Check sheet for the modelled part. Datum: model origin and axes. Units: mm. Face numbers are marked on the shaded views. A direction names the side the tool comes from. Give positions to 0.01 mm unless a question says otherwise; leave off trailing zeros. Order: outer loops, then holes, each group sorted by start corner. A loop starts at its lowest first (then second) coordinate and runs counter-clockwise, first axis right, second up.
Item 1: Sectioned sample at D-D on x = 708. Record the boundary of the cut face in (y, z), and give its area (3 significant figures).
Item 2: Access from +Z, -Z, +X, -X, +Y, -Y to the whole of each face (thin tool, end or side, straight path). Record for the marked faces 1, 2 and 3.
Item 3: Sectioned sample at A-A on x = 144. Record the boundary of the cut face in (y, z), and give its area (3 significant figures).
Item 4: Release check for a two-part mould opening along Y. For the marked faces 4, 5, 6 and 7 record: released by +Y, released by -Y, zero draft, split by the parting line, or undercut.
Item 5: Material ranges on line 1 along Z through (x, y) = (1072, 76) (3 decimals); line 2 along Y through (x, z) = (584.5, 293.5); line 3 along Y through (x, z) = (560, -245.5), recorded low to high.
Item 6: Gauge pin test, flat ends, axial feed: P1, Ø6, axis at x = 123.5, z = 272.5, coming from the +Y side; P2, Ø20.5, axis at x = -667, z = 305.5, coming from the +Y side; P3, Ø6.5, axis at x = 1057.5, z = -48, coming from the +Y side. Record the tip position at first contact, or that the pin passes through.
Item 7: Sectioned sample at B-B on y = 381. Record the boundary of the cut face in (x, z), and give its area (3 significant figures).
Item 8: Sectioned sample at C-C on z = -208. Record the boundary of the cut face in (x, y).
from build123d import *

# Parameters (mm, degrees)
F1_DEPTH  = 1066.8
F2_W      = 101.6
F2_H      = 793.75
F2_R      = 14.2875
F3_DEPTH  = 139.7
F4_W      = 304.8
F4_H      = 222.25
F4_R      = 23.8125
F4_W_2    = 476.25
F5_DEPTH  = 25.4
F8_DEPTH  = 12.7
F9_W      = 101.6
F9_H      = 228.6
F9_R      = 7.14375
F10_DEPTH = 25.4


with BuildPart() as f1:
    # F0 (on Right) → F1 (new body, symmetric)
    with BuildSketch(Plane.YZ):
        with BuildLine():
            Line((476.25, 292.1), (-476.25, 292.1))
            ThreePointArc((-476.25, 292.1), (-498.7006403027, 282.8006403027), (-508, 260.35))
            Line((-508, 260.35), (-508, -260.35))
            ThreePointArc((-508, -260.35), (-513.5796158184, -273.8203841816), (-527.05, -279.4))
            Line((-527.05, -279.4), (-647.7, -279.4))
            Line((-647.7, -279.4), (-647.7, -292.1))
            Line((-647.7, -292.1), (-527.05, -292.1))
            ThreePointArc((-527.05, -292.1), (-504.5993596973, -282.8006403027), (-495.3, -260.35))
            Line((-495.3, -260.35), (-495.3, 260.35))
            ThreePointArc((-495.3, 260.35), (-489.7203841816, 273.8203841816), (-476.25, 279.4))
            Line((-476.25, 279.4), (476.25, 279.4))
            ThreePointArc((476.25, 279.4), (489.7203841816, 273.8203841816), (495.3, 260.35))
            Line((495.3, 260.35), (495.3, -260.35))
            ThreePointArc((495.3, -260.35), (504.5993596973, -282.8006403027), (527.05, -292.1))
            Line((527.05, -292.1), (647.7, -292.1))
            Line((647.7, -292.1), (647.7, -279.4))
            Line((647.7, -279.4), (527.05, -279.4))
            ThreePointArc((527.05, -279.4), (513.5796158184, -273.8203841816), (508, -260.35))
            Line((508, -260.35), (508, 260.35))
            ThreePointArc((508, 260.35), (498.7006403027, 282.8006403027), (476.25, 292.1))
        make_face()
    extrude(amount=F1_DEPTH, both=True)

    # F2 (on face) → F3 (join)
    with BuildSketch(Plane.XY.offset(292.1)):
        with Locations((901.7, -79.375)):
            Rectangle(F2_W, F2_H)
        with Locations((885.952, -234.95)):
            Circle(F2_R, mode=Mode.SUBTRACT)
        with Locations((885.952, 234.95)):
            Circle(F2_R, mode=Mode.SUBTRACT)
        with Locations((565.404, -79.375)):
            Rectangle(F2_W, F2_H)
        with Locations((581.152, -234.95)):
            Circle(F2_R, mode=Mode.SUBTRACT)
        with Locations((581.152, 234.95)):
            Circle(F2_R, mode=Mode.SUBTRACT)
    extrude(amount=F3_DEPTH)

    # F4 (on face) → F5 (join)
    with BuildSketch(Plane.XY.offset(292.1)):
        with Locations((-660.4, -358.775)):
            Rectangle(F4_W, F4_H)
        with Locations((-663.448, -381)):
            Circle(F4_R, mode=Mode.SUBTRACT)
        with Locations((238.125, -358.775)):
            Rectangle(F4_W_2, F4_H)
        with Locations((327.152, -381)):
            Circle(F4_R, mode=Mode.SUBTRACT)
        with Locations((238.125, 358.775)):
            Rectangle(F4_W_2, F4_H)
        with Locations((327.152, 381)):
            Circle(F4_R, mode=Mode.SUBTRACT)
        with Locations((-660.4, 358.775)):
            Rectangle(F4_W, F4_H)
        with Locations((-663.448, 381)):
            Circle(F4_R, mode=Mode.SUBTRACT)
    extrude(amount=F5_DEPTH)

    # F7 (on offset) → F8 (join)
    with BuildSketch(Plane.YZ.offset(1041.4)):
        Polygon((495.3, -260.35), (495.3, 260.35), (476.25, 279.4), (-476.25, 279.4), (-495.3, 260.35), (-495.3, -260.35), align=None)
    extrude(amount=F8_DEPTH)

    # F9 (on face) → F10 (join)
    with BuildSketch(Plane.YZ.offset(1054.1)):
        with Locations((50.8, 136.525)):
            Rectangle(F9_W, F9_H)
        with Locations((76.2, 85.852)):
            Circle(F9_R, mode=Mode.SUBTRACT)
        with Locations((76.2, 212.852)):
            Circle(F9_R, mode=Mode.SUBTRACT)
        with Locations((-50.8, 136.525)):
            Rectangle(F9_W, F9_H)
        with Locations((-76.2, 85.852)):
            Circle(F9_R, mode=Mode.SUBTRACT)
        with Locations((-76.2, 212.852)):
            Circle(F9_R, mode=Mode.SUBTRACT)
    extrude(amount=F10_DEPTH)


solid = f1.part
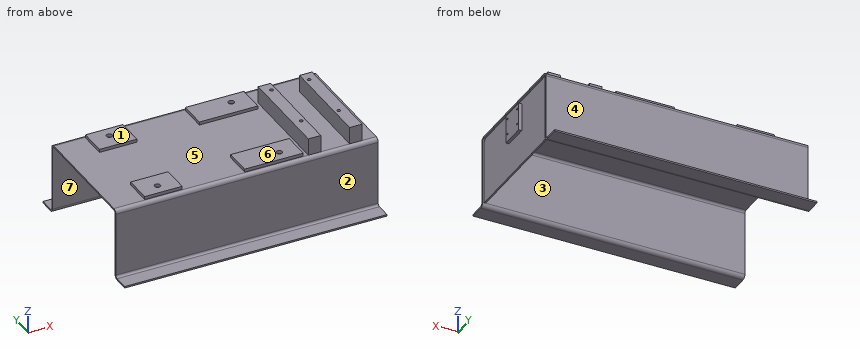
Report:
1. outline: (-647.7, -292.1) - (-527.05, -292.1) arc R31.75 ccw to (-495.3, -260.35) - (-495.3, 260.35) arc R19.05 cw to (-476.25, 279.4) - (476.25, 279.4) arc R19.05 cw to (495.3, 260.35) - (495.3, -260.35) arc R31.75 ccw to (527.05, -292.1) - (647.7, -292.1) - (647.7, -279.4) - (527.05, -279.4) arc R19.05 cw to (508, -260.35) - (508, 260.35) arc R31.75 ccw to (476.25, 292.1) - (-476.25, 292.1) arc R31.75 ccw to (-508, 260.35) - (-508, -260.35) arc R19.05 cw to (-527.05, -279.4) - (-647.7, -279.4) - close
1. area: 30,400 mm2
2. face 1: +Z, -X, +Y, -Y
2. face 2: +Z, +X, -X, -Y
2. face 3: -Z, -X
3. outline: (-647.7, -292.1) - (-527.05, -292.1) arc R31.75 ccw to (-495.3, -260.35) - (-495.3, 260.35) arc R19.05 cw to (-476.25, 279.4) - (476.25, 279.4) arc R19.05 cw to (495.3, 260.35) - (495.3, -260.35) arc R31.75 ccw to (527.05, -292.1) - (647.7, -292.1) - (647.7, -279.4) - (527.05, -279.4) arc R19.05 cw to (508, -260.35) - (508, 260.35) arc R31.75 ccw to (476.25, 292.1) - (469.9, 292.1) - (469.9, 317.5) - (247.65, 317.5) - (247.65, 292.1) - (-247.65, 292.1) - (-247.65, 317.5) - (-469.9, 317.5) - (-469.9, 292.1) - (-476.25, 292.1) arc R31.75 ccw to (-508, 260.35) - (-508, -260.35) arc R19.05 cw to (-527.05, -279.4) - (-647.7, -279.4) - close
3. area: 41,700 mm2
4. face 4: released by +Y
4. face 5: undercut
4. face 6: zero draft
4. face 7: undercut
5. line 1: z = 22.225 to 78.711, 92.993 to 205.711, 219.993 to 250.825
5. line 2: y = -476.25 to -248.84, -221.06 to 221.06, 248.84 to 317.5
5. line 3: y = -508 to -495.3, 495.3 to 508
6. P1: stops at y = 506.65
6. P2: stops at y = 469.9
6. P3: stops at y = 508
7. outline: (-1066.8, 279.4) - (1041.4, 279.4) - (1041.4, -260.35) - (1054.1, -260.35) - (1054.1, 279.4) - (1066.8, 279.4) - (1066.8, 292.1) - (476.25, 292.1) - (476.25, 317.5) - (350.96, 317.5) - (350.96, 292.1) - (303.34, 292.1) - (303.34, 317.5) - (0, 317.5) - (0, 292.1) - (-508, 292.1) - (-508, 317.5) - (-639.64, 317.5) - (-639.64, 292.1) - (-687.26, 292.1) - (-687.26, 317.5) - (-812.8, 317.5) - (-812.8, 292.1) - (-1066.8, 292.1) - close
7. area: 51,400 mm2
8. outline: (-1066.8, -508) - (1066.8, -508) - (1066.8, -495.3) - (1054.1, -495.3) - (1054.1, 495.3) - (1066.8, 495.3) - (1066.8, 508) - (-1066.8, 508) - (-1066.8, 495.3) - (1041.4, 495.3) - (1041.4, -495.3) - (-1066.8, -495.3) - close
